Part model, mm, in its own coordinate system. Face numbers are marked on the shaded views. A direction names the side the tool comes from. Give positions to 0.01 mm unless a question says otherwise; leave off trailing zeros. Loops run counter-clockwise (first coordinate to the right, second up) from the corner with the lowest first, then second, coordinate; pieces in that order, holes last. Notation, with made-up numbers: (12, 50.25) -> (40, 50.25) arc R20 ccw to (40, 83.25) -> close; hole circle Ø3 at (62.5, -12.5). An arc over 180 degrees is marked (long way). One line per question, with ' | ' between items.
```python
from build123d import *

# Parameters (mm, degrees)
F0_W             = 120
F0_H             = 120
F1_DEPTH         = 1.5
F5_W             = 120
F5_H             = 120
F5_W_2           = 112
F5_H_2           = 112
F6_DEPTH         = 1.5
F4_W             = 24
F4_H             = 24
F7_DEPTH         = 1.5
F7_COPIES_COUNT  = 4
F2_W             = 20
F2_H             = 20
F8_DEPTH         = 1.5
F8_COPIES_COUNT  = 4
F10_DEPTH        = 1.5
F12_DEPTH        = 1.5
F12_COPIES_COUNT = 4
F14_DEPTH        = 1.5
F14_COPIES_COUNT = 4
F16_R            = 1.6
F17_DEPTH        = 1.5


# Not quite as in the source:
# - a pattern or mirror of a feature is missing from the dataset's text; its kind, count and spacing are read off the source's solid


with BuildPart() as f1:
    # F0 (on Top) → F1 (new body)
    with BuildSketch(Plane.XY):
        Rectangle(F0_W, F0_H)
    extrude(amount=F1_DEPTH)

    # F5 (on face) → F6 (join)
    with BuildSketch(Plane(origin=(0, 0, 0), x_dir=(1, 0, 0), z_dir=(0, 0, -1))):
        Rectangle(F5_W, F5_H)
        Rectangle(F5_W_2, F5_H_2, mode=Mode.SUBTRACT)
    extrude(amount=F6_DEPTH)

    # F4 (on face) → F7 (join)
    with BuildSketch(Plane(origin=(0, 0, 0), x_dir=(1, 0, 0), z_dir=(0, 0, -1))):
        with Locations((0, -46)):
            Rectangle(F4_W, F4_H)
    f7 = extrude(amount=F7_DEPTH)

    # F7_copies: F7 ×4 about axis
    f7_copies_axis = Axis((0, 0, 0), (0, 0, 1))
    for i in range(1, F7_COPIES_COUNT):
        add(f7.rotate(f7_copies_axis, i * 360 / F7_COPIES_COUNT))

    # F2 (on face) → F8 (cut)
    with BuildSketch(Plane.XY.offset(1.5)):
        with Locations((0, 46)):
            Rectangle(F2_W, F2_H)
    f8 = extrude(amount=-F8_DEPTH, mode=Mode.SUBTRACT)

    # F8_copies: F8 ×4 about axis
    f8_copies_axis = Axis((0, 0, 0), (0, 0, 1))
    for i in range(1, F8_COPIES_COUNT):
        add(f8.rotate(f8_copies_axis, i * 360 / F8_COPIES_COUNT), mode=Mode.SUBTRACT)

    # F9 (on face) → F10 (join)
    with BuildSketch(Plane(origin=(0, 0, 0), x_dir=(1, 0, 0), z_dir=(0, 0, -1))):
        Polygon((-56, 56), (-56, 53.1715728753), (53.1715728753, -56), (56, -56), (56, -53.1715728753), (-53.1715728753, 56), align=None)
    f10 = extrude(amount=F10_DEPTH)

    # F10_copies: F10 across plane
    add(f10.mirror(Plane(origin=(0, 0, 0), x_dir=(0, 0, -1), z_dir=(-1, 0, 0))))

    # F11 (on face) → F12 (join)
    with BuildSketch(Plane(origin=(0, 0, 0), x_dir=(1, 0, 0), z_dir=(0, 0, -1))):
        Polygon((34, 9.1715728753), (34, 12), (36.8284271247, 12), (25.8284271247, 23), (23, 20.1715728753), align=None)
    f12 = extrude(amount=F12_DEPTH)

    # F12_copies: F12 ×4 about axis
    f12_copies_axis = Axis((0, 0, 0), (0, 0, 1))
    for i in range(1, F12_COPIES_COUNT):
        add(f12.rotate(f12_copies_axis, i * 360 / F12_COPIES_COUNT))

    # F13 (on face) → F14 (join)
    with BuildSketch(Plane(origin=(0, 0, 0), x_dir=(1, 0, 0), z_dir=(0, 0, -1))):
        Polygon((12, 36.8284271247), (12, 34), (9.1715728753, 34), (20.1715728753, 23), (23, 25.8284271247), align=None)
    f14 = extrude(amount=F14_DEPTH)

    # F14_copies: F14 ×4 about axis
    f14_copies_axis = Axis((0, 0, 0), (0, 0, 1))
    for i in range(1, F14_COPIES_COUNT):
        add(f14.rotate(f14_copies_axis, i * 360 / F14_COPIES_COUNT))

    # F16 (on face) → F17 (cut)
    with BuildSketch(Plane.XY.offset(1.5)):
        with Locations((18.25, 4)):
            Circle(F16_R)
        with Locations((18.25, -4)):
            Circle(F16_R)
        with Locations((-18.25, -4)):
            Circle(F16_R)
        with Locations((-18.25, 4)):
            Circle(F16_R)
    extrude(amount=-F17_DEPTH, mode=Mode.SUBTRACT)


solid = f1.part
```
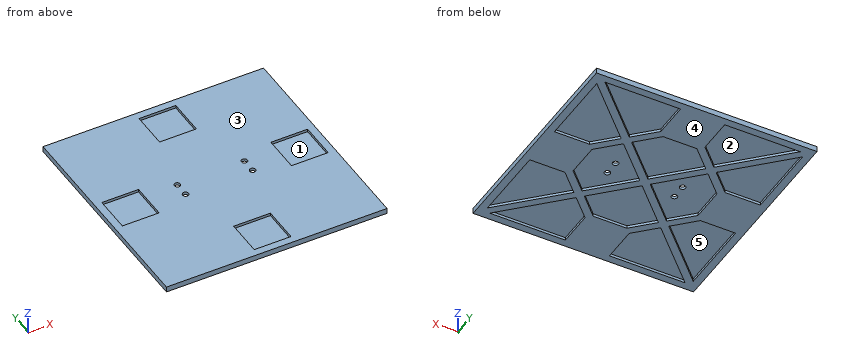
1) Drill centre lines: line 1 (Y direction, x = 4, z = 1.35); line 2 (Y direction, x = -18.25, z = 1.15); line 3 (Y direction, x = 42, z = 0.7). Where is each one in solid material? Low to high.
Found:
line 1: -60 to -56, -36 to 36, 56 to 60 | line 2: -60 to -5.6, -2.4 to 2.4, 5.6 to 60 | line 3: -60 to -10, 10 to 60
2) Pull direction Y, two halves, no side cores. Call the marked faces 4 and 5: pulls with the +Y half, pulls with the -Y half, needs draft (parallel to the pull), parting line crosses it, or undercut.
Found:
face 4: needs draft | face 5: undercut
3) Saw through at A-A (x = 18.25). State how many separate pieces and enclosed holes the cut face has, and give its area (3 significant figures).
Found:
separate pieces: 3 | enclosed holes: 0 | area: 216 mm2
4) Pin check, flat tips, straight feed: P1, Ø8, axis at x = 47.5, y = 5.5, coming from the +Z side; P2, Ø5, axis at x = 18.25, y = 4, coming from the -Z side; P3, Ø3, axis at x = -18.25, y = -4, coming from the -Z side. Stop position of each tip, or through.
Found:
P1: z = 0 | P2: z = 0 | P3: through
5) Tool access for the marked faces 1, 2 and 3: list every direction of +Z, -Z, +X, -X, +Y, -Y with a clear straight run to the whole face (end or side of a thin tool).
Found:
face 1: +Z | face 2: -Z | face 3: +Z, +X, -X, +Y, -Y
6) Saw through at B-B (x = -40.5). Give the cut face in (y, z).
Found:
outline: (-60, -1.5) -> (-56, -1.5) -> (-56, 0) -> (-43.33, 0) -> (-43.33, -1.5) -> (-37.67, -1.5) -> (-37.67, 0) -> (-12, 0) -> (-12, -1.5) -> (12, -1.5) -> (12, 0) -> (37.67, 0) -> (37.67, -1.5) -> (43.33, -1.5) -> (43.33, 0) -> (56, 0) -> (56, -1.5) -> (60, -1.5) -> (60, 1.5) -> (10, 1.5) -> (10, 0) -> (-10, 0) -> (-10, 1.5) -> (-60, 1.5) -> close
